```python
from build123d import *

# Parameters (mm, degrees)
SKETCH1_R           = 4.765
SKETCH1_R_2         = 2
BOSS_EXTRUDE1_DEPTH = 7.5
CUT_EXTRUDE1_START  = -7.5
SKETCH3_R           = 7.765
SKETCH3_W           = 17
SKETCH3_H           = 3.1
CUT_EXTRUDE1_DEPTH  = 7.5


with BuildPart() as part:
    # Sketch1 → Boss-Extrude1 (new body)
    with BuildSketch(Plane.XY):
        with BuildLine():
            Line((-10.765, 32.5), (10.765, 32.5))
            Line((10.765, 32.5), (10.765, -32.5))
            ThreePointArc((10.765, -32.5), (0, -43.265), (-10.765, -32.5))
            Line((-10.765, -32.5), (-10.765, 32.5))
        make_face()
        with Locations((0, -32.5)):
            Circle(SKETCH1_R, mode=Mode.SUBTRACT)
        with Locations((0, 17.835)):
            Circle(SKETCH1_R_2, mode=Mode.SUBTRACT)
        with Locations(Location((0, -12.165, 0), (0, 0, 180))):
            Circle(SKETCH1_R_2, mode=Mode.SUBTRACT)
    extrude(amount=BOSS_EXTRUDE1_DEPTH)

    # Sketch3 → Cut-Extrude1 (cut)
    with BuildSketch(Plane.XY.offset(7.5).offset(CUT_EXTRUDE1_START)):
        with Locations((0, -32.5)):
            Circle(SKETCH3_R)
        Polygon((-5.592339376, -25.913784068), (-2.907660624, -24.363784068), (5.592339376, -39.086215932), (2.907660624, -40.636215932), align=None)
        with Locations((0, -32.5)):
            Rectangle(SKETCH3_W, SKETCH3_H)
        Polygon((2.907660624, -24.363784068), (5.592339376, -25.913784068), (-2.907660624, -40.636215932), (-5.592339376, -39.086215932), align=None)
    extrude(amount=CUT_EXTRUDE1_DEPTH, mode=Mode.SUBTRACT)


solid = part.part
```
Design review of the part built by this model. Coordinates are the model's own, in mm. A direction names the side the tool comes from. Give positions to 0.01 mm unless a question says otherwise; leave off trailing zeros. Order: outer loops, then holes, each group sorted by start corner. A loop starts at its lowest first (then second) coordinate and runs counter-clockwise, first axis right, second up. Notation, with made-up numbers: (61, 22.5) -> (85, 22.5) arc R18 ccw to (85, 50.5) -> close; hole circle Ø3 at (-39.75, -25). An arc over 180 degrees is marked (long way). Write each question's results on one line, items separated by ' | '. Start each with the question number.
Q1. Mouldability with a two-part tool opening along Y and no side actions: class faces 1 (the flat face through (-10.765, 0, 4)), 2 (the cylindrical face through (6.742, -28.648, 3.698)), 3 (the flat face through (0, 32.5, 4)) as +Y half, -Y half, draft (parallel to the pull), parting line (faces both ways), or undercut.
Q2. Wall thickness on L1, parallel to Y at x = 0.25, z = 1.25; L2, parallel to Y at x = -1.5, z = 4.5; L3, parallel to X at y = -32, z = 7.25 (3 decimals): over which ranges is each line inside the solid? List them lowest first. Write a range as from..to.
Q3. Add section C-C on z = 4.5. State how many separate pieces and enclosed holes the cut face has, and give its area (3 significant figures).
Q4. For pin 1 (1.5 mm diameter, centred on x = 3.5, z = 6, fed in from -Y); pin 2 (0.7 mm diameter, centred on x = 8, z = 2, fed in from -Y), all flat-tipped, find the tip position at first contact; note any pin that passes through.
Q5. Machinability: for faces 4 (the flat face through (0, 4, 7.5)), 5 (the flat face through (-4.27, -25.15, 3.7)), which of the approach directions +Z, -Z, +X, -X, +Y, -Y give a long, thin tool a straight path to every point of the face, cutting with its end or side? Answer none if there is none.
Q6. Add section B-B on y = -36.5. Give the boundary of the cut face in (x, z).
Q7. Add section D-D on x = -3.75. Give the boundary of the cut face in (y, z), and give its area (3 significant figures).
Q8. Add section A-A on x = 0. Give the boundary of the cut face in (y, z) (3 decimals).
Found:
1) face 1: draft | face 2: undercut | face 3: +Y half
2) L1: y = -43.26..-40.26, -24.74..-14.15, -10.18..15.85, 19.82..32.5 | L2: y = -43.16..-40.12, -24.88..-13.49, -10.84..16.51, 19.16..32.5 | L3: x = -10.765..-8.5, 8.5..10.765
3) separate pieces: 1 | enclosed holes: 3 | area: 1,350 mm2
4) pin 1: stops at y = -42.91 | pin 2: stops at y = -40.07
5) face 4: +Z, +X, -X, +Y, -Y | face 5: +Z, -Z
6) outline: (-9.99, 0) -> (-6.66, 0) -> (-6.66, 7.5) -> (-9.99, 7.5) -> close; (6.66, 0) -> (9.99, 0) -> (9.99, 7.5) -> (6.66, 7.5) -> close
7) outline: (-42.59, 0) -> (-40.15, 0) -> (-40.15, 7.5) -> (-42.59, 7.5) -> close; (-24.85, 0) -> (32.5, 0) -> (32.5, 7.5) -> (-24.85, 7.5) -> close | area: 448 mm2
8) outline: (-43.265, 0) -> (-40.265, 0) -> (-40.265, 7.5) -> (-43.265, 7.5) -> close; (-24.735, 0) -> (-14.165, 0) -> (-14.165, 7.5) -> (-24.735, 7.5) -> close; (-10.165, 0) -> (15.835, 0) -> (15.835, 7.5) -> (-10.165, 7.5) -> close; (19.835, 0) -> (32.5, 0) -> (32.5, 7.5) -> (19.835, 7.5) -> close
